```python
from build123d import *

# Parameters (mm, degrees)
F0_R     = 14.2875
F1_DEPTH = 25.146
F2_DEPTH = 26.162


with BuildPart() as f1:
    # F0 (on Front) → F1 (new body)
    with BuildSketch(Plane.XZ):
        with BuildLine():
            Line((9.7116618994, 26.8740441347), (0, 28.575))
            ThreePointArc((0, 28.575), (-28.575, 0), (0, -28.575))
            Line((0, -28.575), (9.6830426125, -26.8843692648))
            ThreePointArc((9.6830426125, -26.8843692648), (23.3797301915, -16.4292069551), (28.575, 0))
            ThreePointArc((28.575, 0), (23.3884732697, 16.4167579964), (9.7116618994, 26.8740441347))
        make_face()
        with BuildLine():
            ThreePointArc((-13.4703841816, 4.7625), (0, 14.2875), (13.4703841816, 4.7625))
            Line((13.4703841816, 4.7625), (19.05, 4.7625))
            Line((19.05, 4.7625), (19.05, -4.7625))
            Line((19.05, -4.7625), (13.4703841816, -4.7625))
            ThreePointArc((13.4703841816, -4.7625), (0, -14.2875), (-13.4703841816, -4.7625))
            Line((-13.4703841816, -4.7625), (-19.05, -4.7625))
            Line((-19.05, -4.7625), (-19.05, 4.7625))
            Line((-19.05, 4.7625), (-13.4703841816, 4.7625))
        make_face(mode=Mode.SUBTRACT)
        with BuildLine():
            Line((54.4119007606, 19.0449893076), (9.7116618994, 26.8740441347))
            ThreePointArc((9.7116618994, 26.8740441347), (23.3884732697, 16.4167579964), (28.575, 0))
            ThreePointArc((28.575, 0), (23.3797301915, -16.4292069551), (9.6830426125, -26.8843692648))
            Line((9.6830426125, -26.8843692648), (54.6159610506, -19.0392139788))
            ThreePointArc((54.6159610506, -19.0392139788), (34.9252734531, -0.1020710003), (54.4119007606, 19.0449893076))
        make_face()
        with BuildLine():
            ThreePointArc((73.025, 0), (67.5989762825, 13.3150204752), (54.4119007606, 19.0449893076))
            ThreePointArc((54.4119007606, 19.0449893076), (34.9252734531, -0.1020710003), (54.6159610506, -19.0392139788))
            ThreePointArc((54.6159610506, -19.0392139788), (67.6701233659, -13.241831293), (73.025, 0))
        make_face()
        with Locations((53.975, 0)):
            Circle(F0_R, mode=Mode.SUBTRACT)
        with BuildLine():
            ThreePointArc((-13.4703841816, -4.7625), (-14.2875, 0), (-13.4703841816, 4.7625))
            Line((-13.4703841816, 4.7625), (-19.05, 4.7625))
            Line((-19.05, 4.7625), (-19.05, -4.7625))
            Line((-19.05, -4.7625), (-13.4703841816, -4.7625))
        make_face()
    extrude(amount=F1_DEPTH)

    # F0 (on Front) → F2 (join)
    with BuildSketch(Plane.XZ):
        with BuildLine():
            Line((9.7116618994, 26.8740441347), (0, 28.575))
            ThreePointArc((0, 28.575), (-28.575, 0), (0, -28.575))
            Line((0, -28.575), (9.6830426125, -26.8843692648))
            ThreePointArc((9.6830426125, -26.8843692648), (23.3797301915, -16.4292069551), (28.575, 0))
            ThreePointArc((28.575, 0), (23.3884732697, 16.4167579964), (9.7116618994, 26.8740441347))
        make_face()
        with BuildLine():
            ThreePointArc((-13.4703841816, 4.7625), (0, 14.2875), (13.4703841816, 4.7625))
            Line((13.4703841816, 4.7625), (19.05, 4.7625))
            Line((19.05, 4.7625), (19.05, -4.7625))
            Line((19.05, -4.7625), (13.4703841816, -4.7625))
            ThreePointArc((13.4703841816, -4.7625), (0, -14.2875), (-13.4703841816, -4.7625))
            Line((-13.4703841816, -4.7625), (-19.05, -4.7625))
            Line((-19.05, -4.7625), (-19.05, 4.7625))
            Line((-19.05, 4.7625), (-13.4703841816, 4.7625))
        make_face(mode=Mode.SUBTRACT)
        with BuildLine():
            ThreePointArc((-13.4703841816, -4.7625), (-14.2875, 0), (-13.4703841816, 4.7625))
            Line((-13.4703841816, 4.7625), (-19.05, 4.7625))
            Line((-19.05, 4.7625), (-19.05, -4.7625))
            Line((-19.05, -4.7625), (-13.4703841816, -4.7625))
        make_face()
    extrude(amount=-F2_DEPTH)


solid = f1.part
```
Input: part model. Units: mm. Frame: model coordinates. A direction names the side the tool comes from. Give positions to 0.01 mm unless a question says otherwise; leave off trailing zeros. Order: outer loops, then holes, each group sorted by start corner. A loop starts at its lowest first (then second) coordinate and runs counter-clockwise, first axis right, second up.
1. Cut plane C-C (x = 50). Return loops of the section in (y, z).
Computed:
outline: (-25.15, -19.85) - (0, -19.85) - (0, -13.72) - (-25.15, -13.72) - close; (-25.15, 13.72) - (0, 13.72) - (0, 19.82) - (-25.15, 19.82) - close
2. Pin query (flat end, axial travel): pin 1 Ø12 at (x, y) = (57.5, -18) entering from +Z (3 decimals); pin 2 Ø5 at (y, z) = (-11, -1.5) entering from -X (3 decimals); pin 3 Ø2 at (x, y) = (3, 9) entering from +Z. Return the tip coordinate at first contact, or that it passes through.
Computed:
pin 1: stops at z = 19.555
pin 2: stops at x = -28.575
pin 3: stops at z = 28.22
3. Line query: probe 1 along X at (y, z) = (-13.5, -10); probe 2 along X at (y, z) = (-12, -11); probe 3 along X at (y, z) = (20, 8). Output: solid intervals per line, ascending.
Computed:
probe 1: x = -26.77 to -10.2, 10.2 to 43.77, 64.18 to 70.19
probe 2: x = -26.37 to -9.12, 9.12 to 44.86, 63.09 to 69.53
probe 3: x = -27.43 to -11.84, 11.84 to 27.43
4. Set-up query: faces 1 (the face through (16, 0, 4.762)), 2 (the face through (22, -25.146, 0)). Return all of +Z, -Z, +X, -X, +Y, -Y with unobstructed straight access to the full face (end or side cutting, diameter ignored); none if empty.
Computed:
face 1: +Y, -Y
face 2: +Z, -Z, +X, -X, -Y
5. Cut plane B-B (z = 9.5). Return loops of the section in (x, y), and give its area (3 significant figures).
Computed:
outline: (-26.95, -25.15) - (-10.67, -25.15) - (-10.67, 26.16) - (-26.95, 26.16) - close; (10.67, -25.15) - (43.3, -25.15) - (43.3, 0) - (26.95, 0) - (26.95, 26.16) - (10.67, 26.16) - close; (64.65, -25.15) - (70.49, -25.15) - (70.49, 0) - (64.65, 0) - close
area: 2,230 mm2
6. Cut plane D-D (y = -4.5). State how many separate pieces and enclosed holes the cut face has, and give its area (3 significant figures).
Computed:
separate pieces: 1
enclosed holes: 2
area: 3,100 mm2
7. Draft query along X for faces 3 (the face through (39, 0, -2)), 4 (the face through (-28.57, 0.15, 0.63)), 5 (the face through (67.6, -12.4, 4.3)), 6 (the face through (28.57, 12.9, -0.51)). Return one class per face: released by +X, released by -X, zero draft, split by the parting line, or undercut.
Computed:
face 3: zero draft
face 4: released by -X
face 5: undercut
face 6: released by +X
